from build123d import *

# Parameters (mm, degrees)
SKETCH1_W           = 600
SKETCH1_H           = 60
BOSS_EXTRUDE1_DEPTH = 3
SKETCH4_W           = 600
SKETCH4_H           = 60
BOSS_EXTRUDE4_DEPTH = 3
SKETCH2_W           = 30
SKETCH2_H           = 3
SKETCH2_W_2         = 3
SKETCH2_H_2         = 30
CUT_EXTRUDE1_DEPTH  = 5
SKETCH5_W           = 167
SKETCH5_H           = 49
CUT_EXTRUDE2_DEPTH  = 5
CUT_EXTRUDE3_DEPTH  = 5


with BuildPart() as part:
    # Sketch1 → Boss-Extrude1 (new body)
    with BuildSketch(Plane(origin=(0, 0, 0), x_dir=(1, 0, 0), z_dir=(0, 1, 0))):
        with Locations((300, 30)):
            Rectangle(SKETCH1_W, SKETCH1_H)
    extrude(amount=BOSS_EXTRUDE1_DEPTH)

    # Sketch4 → Boss-Extrude4 (add)
    with BuildSketch(Plane(origin=(0, 3, 0), x_dir=(1, 0, 0), z_dir=(0, 1, 0))):
        with Locations((300, -30)):
            Rectangle(SKETCH4_W, SKETCH4_H)
    extrude(amount=-BOSS_EXTRUDE4_DEPTH)

    # Sketch2 → Cut-Extrude1 (cut)
    with BuildSketch(Plane(origin=(0, 3, 0), x_dir=(1, 0, 0), z_dir=(0, 1, 0))):
        with Locations((0, 1.5)):
            Rectangle(SKETCH2_W, SKETCH2_H)
        with Locations((60, 1.5)):
            Rectangle(SKETCH2_W, SKETCH2_H)
        with Locations((120, 1.5)):
            Rectangle(SKETCH2_W, SKETCH2_H)
        with Locations((180, 1.5)):
            Rectangle(SKETCH2_W, SKETCH2_H)
        with Locations((240, 1.5)):
            Rectangle(SKETCH2_W, SKETCH2_H)
        with Locations((300, 1.5)):
            Rectangle(SKETCH2_W, SKETCH2_H)
        with Locations((360, 1.5)):
            Rectangle(SKETCH2_W, SKETCH2_H)
        with Locations((420, 1.5)):
            Rectangle(SKETCH2_W, SKETCH2_H)
        with Locations((480, 1.5)):
            Rectangle(SKETCH2_W, SKETCH2_H)
        with Locations((540, 1.5)):
            Rectangle(SKETCH2_W, SKETCH2_H)
        with Locations((598.5, 30)):
            Rectangle(SKETCH2_W_2, SKETCH2_H_2)
        with Locations((540, 58.5)):
            Rectangle(SKETCH2_W, SKETCH2_H)
        with Locations((480, 58.5)):
            Rectangle(SKETCH2_W, SKETCH2_H)
        with Locations((420, 58.5)):
            Rectangle(SKETCH2_W, SKETCH2_H)
        with Locations((360, 58.5)):
            Rectangle(SKETCH2_W, SKETCH2_H)
        with Locations((300, 58.5)):
            Rectangle(SKETCH2_W, SKETCH2_H)
        with Locations((240, 58.5)):
            Rectangle(SKETCH2_W, SKETCH2_H)
        with Locations((180, 58.5)):
            Rectangle(SKETCH2_W, SKETCH2_H)
        with Locations((120, 58.5)):
            Rectangle(SKETCH2_W, SKETCH2_H)
        with Locations((60, 58.5)):
            Rectangle(SKETCH2_W, SKETCH2_H)
        with Locations((0, 58.5)):
            Rectangle(SKETCH2_W, SKETCH2_H)
        with Locations((1.5, 30)):
            Rectangle(SKETCH2_W_2, SKETCH2_H_2)
        with Locations((600, 1.5)):
            Rectangle(SKETCH2_W, SKETCH2_H)
        with Locations((600, 58.5)):
            Rectangle(SKETCH2_W, SKETCH2_H)
    extrude(amount=-CUT_EXTRUDE1_DEPTH, mode=Mode.SUBTRACT)

    # Sketch5 → Cut-Extrude2 (cut)
    with BuildSketch(Plane(origin=(0, 3, 0), x_dir=(1, 0, 0), z_dir=(0, 1, 0))):
        with Locations((300, 27.5)):
            Rectangle(SKETCH5_W, SKETCH5_H)
    extrude(amount=-CUT_EXTRUDE2_DEPTH, mode=Mode.SUBTRACT)

    # Sketch6 → Cut-Extrude3 (cut)
    with BuildSketch(Plane(origin=(0, 3, 0), x_dir=(1, 0, 0), z_dir=(0, 1, 0))):
        with BuildLine():
            Line((80, -60), (520, -60))
            ThreePointArc((520, -60), (300, -20), (80, -60))
        make_face()
    extrude(amount=-CUT_EXTRUDE3_DEPTH, mode=Mode.SUBTRACT)


solid = part.part
Could you check a few things on this model? Use its own coordinates, in mm. Give positions to 0.01 mm unless a question says otherwise; leave off trailing zeros. Order: outer loops, then holes, each group sorted by start corner. A loop starts at its lowest first (then second) coordinate and runs counter-clockwise, first axis right, second up. Notation, with made-up numbers: (48, -12.75) - (104, -12.75) arc R11 cw to (104, -0.75) - close; hole circle Ø5 at (55.25, -1.75). An arc over 180 degrees is marked (long way). One line per item, written item: value. Start each with the question number.
1. Imagine slicing it at A-A on z = -20.5. List the corners of the cut face in (x, y) for me.
2. Imagine slicing it at C-C on y = 1. Give the number of separate pieces and of enclosed holes in the cut face, plus the area to 3 significant figures.
3. Imagine slicing it at B-B on x = 471. List the corners of the cut face in (y, z) for me, plus the area to 3 significant figures.
4. Imagine slicing it at D-D on x = 100. List the corners of the cut face in (y, z) for me, plus the area to 3 significant figures.
5. For P1, Ø1.5, axis at x = 185, y = 1.5, coming from the +Z side; P2, Ø1.5, axis at y = 1.5, z = -58.5, coming from the +X side; P3, Ø1.5, axis at x = 483, y = 1, coming from the -Z side, each with a flat end and sliding along its axis, tell me the tip position at first contact or that it passes through.
6. If I drill on probe 1 along Z at (x, y) = (304, 0.3); probe 2 along X at (y, z) = (0.2, -32); probe 3 along X at (y, z) = (0.7, -47), over which ranges is the centre line in solid material (lowest first)?
7. Thinking about a two-plate mould opening in X: for faces 1 (the face through (303.147, 1.521, 20.008)), 2 (the face through (296, 3, 12)), which applies, +X half, -X half, draft (parallel to the pull), parting line (faces both ways), or undercut?
Values:
1. outline: (3, 0) - (216.5, 0) - (216.5, 3) - (3, 3) - close; (383.5, 0) - (597, 0) - (597, 3) - (383.5, 3) - close
2. separate pieces: 1
2. enclosed holes: 7
2. area: 50,000 mm²
3. outline: (0, -57) - (3, -57) - (3, -3) - (0, -3) - close; (0, 0) - (3, 0) - (3, 43.85) - (0, 43.85) - close
3. area: 294 mm²
4. outline: (0, -60) - (3, -60) - (3, 52.86) - (0, 52.86) - close
4. area: 339 mm²
5. P1: z = 30.81
5. P2: x = 585
5. P3: z = -57
6. probe 1: -57 to -52, 0 to 20.01
6. probe 2: 3 to 216.5, 383.5 to 597
6. probe 3: 0 to 216.5, 383.5 to 600
7. face 1: undercut
7. face 2: draft
